Design review of the part built by this model. Coordinates are the model's own, in mm. Coordinates: 2 decimals unless noted, no trailing zeros. Write each loop counter-clockwise with the first axis right and the second up, starting at its lowest first coordinate (ties: lowest second). Pieces come first, ordered by that corner, then holes. Notation, with made-up numbers: (-22, 68) - (-6, 68) arc R23 cw to (-6, 81) - close; hole circle Ø11 at (18, 0). An arc over 180 degrees is marked (long way). Use a Markdown table: item, result.
from build123d import *

# Parameters (mm, degrees)
F0_W     = 50.8
F0_H     = 101.6
F0_R     = 7.62
F1_DEPTH = 12.7
F2_R     = 5.08
F3_R     = 4.529312
F4_DEPTH = 25.4


with BuildPart() as f1:
    # F0 (on Front) → F1 (new body, symmetric)
    with BuildSketch(Plane.XZ):
        Rectangle(F0_W, F0_H)
        with Locations((0, -27.454738)):
            Circle(F0_R, mode=Mode.SUBTRACT)
        with Locations((0, 27.454738)):
            Circle(F0_R, mode=Mode.SUBTRACT)
    extrude(amount=F1_DEPTH, both=True)

    # F2
    f2_edges = [f1.edges().sort_by_distance(p)[0] for p in [
        (25.4, 0, 50.8),
        (-25.4, 0, 50.8),
        (-25.4, 0, -50.8),
        (25.4, 0, -50.8),
    ]]
    fillet(f2_edges, radius=F2_R)

    # F3 (on face) → F4 (cut, through all)
    with BuildSketch(Plane.XZ.offset(12.7)):
        with Locations((-16.305836, 41.625459)):
            Circle(F3_R)
        with Locations((16.305836, 41.625459)):
            Circle(F3_R)
        with Locations((-16.305836, -41.625459)):
            Circle(F3_R)
        with Locations((16.305836, -41.625459)):
            Circle(F3_R)
    extrude(amount=-F4_DEPTH, mode=Mode.SUBTRACT)


solid = f1.part
(1) Draft analysis for pull direction X (two halves, no side actions). For faces 1 (the cylindrical face through (23.951, 0.178, 49.272)), 2 (the cylindrical face through (-17.288, -0.178, -46.047)), 3 (the cylindrical face through (-23.951, -0.178, -49.272)), 4 (the cylindrical face through (15.716, -0.178, 46.116)), state which applies: +X half, -X half, draft (parallel to the pull), parting line (faces both ways), or undercut.
Determined:
| item | result |
|---|---|
| face 1 | +X half |
| face 2 | undercut |
| face 3 | -X half |
| face 4 | undercut |
(2) Take a section at C-C on y = -2.75. Write out the cut boundary in (x, z), and give its area (3 significant figures).
Determined:
| item | result |
|---|---|
| outline | (-25.4, -45.72) arc R5.08 ccw to (-20.32, -50.8) - (20.32, -50.8) arc R5.08 ccw to (25.4, -45.72) - (25.4, 45.72) arc R5.08 ccw to (20.32, 50.8) - (-20.32, 50.8) arc R5.08 ccw to (-25.4, 45.72) - close; hole circle Ø9.06 at (-16.31, -41.63); hole circle Ø9.06 at (-16.31, 41.63); hole circle Ø15.24 at (0, -27.45); hole circle Ø15.24 at (0, 27.45); hole circle Ø9.06 at (16.31, -41.63); hole circle Ø9.06 at (16.31, 41.63) |
| area | 4,520 mm2 |
(3) Take a section at D-D on z = -31. Write out the cut boundary in (x, y).
Determined:
| item | result |
|---|---|
| outline | (-25.4, -12.7) - (-6.75, -12.7) - (-6.75, 12.7) - (-25.4, 12.7) - close; (6.75, -12.7) - (25.4, -12.7) - (25.4, 12.7) - (6.75, 12.7) - close |
(4) For L1, parallel to Z at x = 0, y = 0; L2, parallel to Z at x = -17, y = -3; L3, parallel to X at y = 11.25, z = 40, list the stretches that pass through material, from the lowest coordinate up. Write a range as from..to.
Determined:
| item | result |
|---|---|
| L1 | -50.8..-35.07, -19.83..19.83, 35.07..50.8 |
| L2 | -50.8..-46.1, -37.15..37.15, 46.1..50.8 |
| L3 | -25.4..-20.53, -12.08..12.08, 20.53..25.4 |
(5) Take a section at A-A on x = 0. Write out the cut boundary in (y, z), and give its area (3 significant figures).
Determined:
| item | result |
|---|---|
| outline | (-12.7, -50.8) - (12.7, -50.8) - (12.7, -35.07) - (-12.7, -35.07) - close; (-12.7, -19.83) - (12.7, -19.83) - (12.7, 19.83) - (-12.7, 19.83) - close; (-12.7, 35.07) - (12.7, 35.07) - (12.7, 50.8) - (-12.7, 50.8) - close |
| area | 1,810 mm2 |
(6) Take a section at B-B on z = 34. Write out the cut boundary in (x, y).
Determined:
| item | result |
|---|---|
| outline | (-25.4, -12.7) - (-3.9, -12.7) - (-3.9, 12.7) - (-25.4, 12.7) - close; (3.9, -12.7) - (25.4, -12.7) - (25.4, 12.7) - (3.9, 12.7) - close |
